from build123d import *

# Parameters (mm, degrees)
F2_SCALE  = 1.7860860832
F3_SCALE  = 1.2857142857
F5_DEPTH  = 127
F7_R      = 1.9685
F8_DEPTH  = 25.4
F10_COUNT = 6
F12_R     = 3.556
F13_DEPTH = 20.32


with BuildPart() as f1:
    # F0 (on Front) → F1 (revolve)
    with BuildSketch(Plane.XZ):
        with BuildLine():
            add(Edge.make_bspline(
                [(-12.4434078933, -0.2857490592), (-11.6801978814, 1.4455605736), (-10.132303464, 4.9568935924), (-7.6665859487, 9.8852568378), (-2.720582136, 14.9542509408), (0, 14.9542509408)],
                knots=[0, 0, 0, 0, 0.1522053216, 0.308693235, 0.5, 0.5, 0.5, 0.5], degree=3))
            Line((-12.4434078933, -0.2857490592), (0, -0.2857490592))
            Line((0, -0.2857490592), (0, 14.9542509408))
        make_face()
    revolve(axis=Axis((0, 0, 7.3342509408), (0, 0, 1)))


with BuildPart() as f1_1:
    # F2: moved
    add(f1.part.scale(F2_SCALE))


with BuildPart() as f1_2:
    # F3: moved
    add(f1_1.part.scale(F3_SCALE))

    # F4 (on face) → F5 (cut)
    with BuildSketch(Plane(origin=(0, 0, -0.6561931088), x_dir=(1, 0, 0), z_dir=(0, 0, -1))):
        with BuildLine():
            Line((14.2874984997, 24.7466733145), (0, 0))
            Line((0, 0), (-14.2874984997, 24.7466733145))
            ThreePointArc((-14.2874984997, 24.7466733145), (-14.2874984997, -24.7466733145), (28.5749969994, 0))
            ThreePointArc((28.5749969994, 0), (24.7466733145, 14.2874984997), (14.2874984997, 24.7466733145))
        make_face()
    extrude(amount=-F5_DEPTH, mode=Mode.SUBTRACT)

    # F7 (on offset) → F8 (cut)
    with BuildSketch(Plane.XZ.offset(38.1)):
        with Locations((0, 5.6938068912)):
            Circle(F7_R)
    extrude(amount=-F8_DEPTH, mode=Mode.SUBTRACT)


with BuildPart() as f10_1:
    # F10: instance of F1
    add(f1_2.part.rotate(Axis((0, 0, 23.0994801968), (0, 0, 1)), 1 * 360 / F10_COUNT))


with BuildPart() as f10_2:
    # F10: instance of F1
    add(f1_2.part.rotate(Axis((0, 0, 23.0994801968), (0, 0, 1)), 2 * 360 / F10_COUNT))


with BuildPart() as f10_3:
    # F10: instance of F1
    add(f1_2.part.rotate(Axis((0, 0, 23.0994801968), (0, 0, 1)), 3 * 360 / F10_COUNT))


with BuildPart() as f10_4:
    # F10: instance of F1
    add(f1_2.part.rotate(Axis((0, 0, 23.0994801968), (0, 0, 1)), 4 * 360 / F10_COUNT))


with BuildPart() as f10_5:
    # F10: instance of F1
    add(f1_2.part.rotate(Axis((0, 0, 23.0994801968), (0, 0, 1)), 5 * 360 / F10_COUNT))


with BuildPart() as f1_3:
    add(f1_2.part)

    # F11: union F10_2, F10_1, F10_5, F10_3, F10_4
    add(f10_2.part)
    add(f10_1.part)
    add(f10_5.part)
    add(f10_3.part)
    add(f10_4.part)

    # F12 (on face) → F13 (cut)
    with BuildSketch(Plane(origin=(0, 0, -0.6561931088), x_dir=(1, 0, 0), z_dir=(0, 0, -1))):
        Circle(F12_R)
    extrude(amount=-F13_DEPTH, mode=Mode.SUBTRACT)


solid = f1_3.part
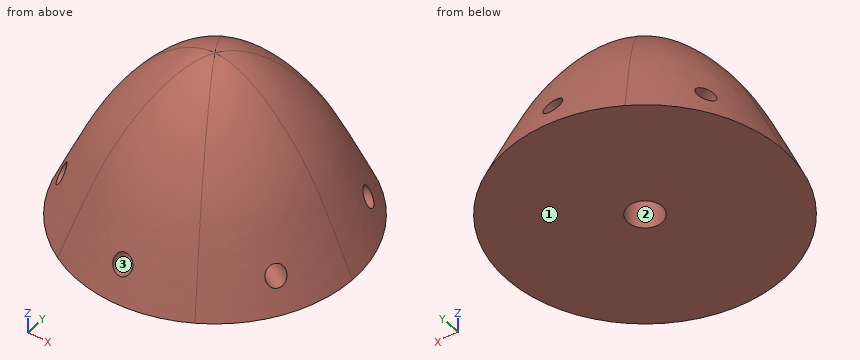
Could you check a few things on this model? Use its own coordinates, in mm. Face numbers are marked on the shaded views. Give positions to 0.01 mm unless a question says otherwise; leave off trailing zeros. Answer as CSV lines item,"result". Start each with the question number.
(1) If we section it at A-A, the plane y = 6.5: Give the number of separate pieces and of enclosed holes in the cut face, and give its area (3 significant figures).
(2) If we mould it in two halves opening along Z, with no side actions, what happens to the marked faces 1, 2 and 3? For each: +Z half, -Z half, draft (parallel to the pull), parting line (faces both ways), or undercut.
(3) I'm going to push flat-ended pins straight in: pin 1 Ø8 at (y, z) = (-5, 19) entering from -X; pin 2 Ø3.5 at (x, z) = (0, 5.69) entering from -Y; pin 3 Ø4 at (x, z) = (6.5, 11.5) entering from +Y. Where does each tip first touch, or does it pass through?
(4) Please list where these lines run through material, in increasing order: line 1 (X direction, y = 9, z = 6); line 2 (Y direction, x = 11, z = 5); line 3 (Y direction, x = 0, z = 4).
Answer list:
1,separate pieces,"1"
1,enclosed holes,"2"
1,area,"1,200 mm^2"
2,face 1,"-Z half"
2,face 2,"draft"
2,face 3,"undercut"
3,pin 1,"x = -20.94"
3,pin 2,"y = -12.7"
3,pin 3,"y = 23.27"
4,line 1,"-23.99 to -19.48, -11.7 to 11.7, 19.48 to 23.99"
4,line 2,"-23.64 to -8.48, -6.35 to 6.35, 8.48 to 23.64"
4,line 3,"-12.7 to -3.56, 3.56 to 12.7"
